from build123d import *

# Parameters (mm, degrees)
SALIENTE_EXTRUIR1_DEPTH = 15
CORTAR_EXTRUIR1_REACH   = 75.655
CROQUIS2_W              = 15
CROQUIS2_H              = 25


with BuildPart() as part:
    # Croquis1 → Saliente-Extruir1 (new, symmetric)
    with BuildSketch(Plane.XY):
        Polygon((-20, 0), (20, 0), (20, 60), (7.5, 60), (7.5, 20), (-7.5, 20), (-7.5, 60), (-20, 60), align=None)
    extrude(amount=SALIENTE_EXTRUIR1_DEPTH, both=True)

    # Croquis2 → Cortar-Extruir1 (cut, up to next)
    with BuildSketch(Plane(origin=(20, 0, 0), x_dir=(0, 0, -1), z_dir=(1, 0, 0)), mode=Mode.PRIVATE) as cortar_extruir1_sk1:
        with Locations((0, 47.5)):
            Rectangle(CROQUIS2_W, CROQUIS2_H)
    cortar_extruir1_tool1 = extrude(cortar_extruir1_sk1.sketch, amount=-CORTAR_EXTRUIR1_REACH, mode=Mode.PRIVATE) & part.part
    cortar_extruir1 = cortar_extruir1_tool1.solids().sort_by_distance((20, 47.5, 0))[0]
    add(cortar_extruir1, mode=Mode.SUBTRACT)

    # Simetría1: Cortar-Extruir1 across plane
    add(cortar_extruir1.mirror(Plane(origin=(0, 0, 0), x_dir=(0, 0, 1), z_dir=(1, 0, 0))), mode=Mode.SUBTRACT)


solid = part.part
The listing builds one solid part. Answer for the finished solid, in the listing's coordinates (mm). A direction names the side the tool comes from. Give positions to 0.01 mm unless a question says otherwise; leave off trailing zeros. Write each loop counter-clockwise with the first axis right and the second up, starting at its lowest first coordinate (ties: lowest second). Pieces come first, ordered by that corner, then holes.
1) Section D-D (y = 52) is taken. Write down the section's boundary in (x, z), and give its area (3 significant figures).
2) Section B-B (z = -11.5) is taken. Write down the section's boundary in (x, y), and give its area (3 significant figures).
3) For a pull along X with two mould halves and no side action, classify faces 4 (the face through (-20, 24, 0)), 5 (the face through (7.5, 31, 0)), 6 (the face through (-14, 47, -7.5)) as pulls with the +X half, pulls with the -X half, needs draft (parallel to the pull), parting line crosses it, or undercut.
4) A tool of negligible diameter and unlimited length cuts with its end or side. For faces 1 (the face through (0, 20, 0)), 2 (the face through (14, 47, 7.5)), 3 (the face through (20, 23, 0)), from which of +Z, -Z, +X, -X, +Y, -Y can it reach the whole face along a straight path? Write none if from no direction.
5) Section C-C (x = -13.5) is taken. Write down the section's boundary in (y, z), and give its area (4 significant figures).
6) Find the intervals of material crossed by L1, parallel to Z at x = 13.5, y = 50.5; L2, parallel to X at y = 27.5, z = -9; L3, parallel to Y at x = -6.5, z = 4.5, in increasing order.
7) Section A-A (y = 24) is taken. Write down the section's boundary in (x, z), and give its area (3 significant figures).
Response:
1. outline: (-20, -15) - (-7.5, -15) - (-7.5, -7.5) - (-20, -7.5) - close; (-20, 7.5) - (-7.5, 7.5) - (-7.5, 15) - (-20, 15) - close; (7.5, -15) - (20, -15) - (20, -7.5) - (7.5, -7.5) - close; (7.5, 7.5) - (20, 7.5) - (20, 15) - (7.5, 15) - close
1. area: 375 mm2
2. outline: (-20, 0) - (20, 0) - (20, 60) - (7.5, 60) - (7.5, 20) - (-7.5, 20) - (-7.5, 60) - (-20, 60) - close
2. area: 1,800 mm2
3. face 4: pulls with the -X half
3. face 5: undercut
3. face 6: needs draft
4. face 1: +Z, -Z, +Y
4. face 2: +X, -X, +Y
4. face 3: +Z, -Z, +X, +Y, -Y
5. outline: (0, -15) - (60, -15) - (60, -7.5) - (35, -7.5) - (35, 7.5) - (60, 7.5) - (60, 15) - (0, 15) - close
5. area: 1,425 mm2
6. L1: z = -15 to -7.5, 7.5 to 15
6. L2: x = -20 to -7.5, 7.5 to 20
6. L3: y = 0 to 20
7. outline: (-20, -15) - (-7.5, -15) - (-7.5, 15) - (-20, 15) - close; (7.5, -15) - (20, -15) - (20, 15) - (7.5, 15) - close
7. area: 750 mm2
